from build123d import *

# Parameters (mm, degrees)
SKETCH1_W         = 247
SKETCH1_H         = 293
MAIN_BASE_DEPTH   = 3.175
HANDLES_DEPTH     = 192.715472772
ALIGNMENT_HOLES_D = 6.99999997


with BuildPart() as part:
    # Sketch1 → Main Base (new, symmetric)
    with BuildSketch(Plane(origin=(0, 0, 0), x_dir=(1, 0, 0), z_dir=(0, 1, 0))):
        Rectangle(SKETCH1_W, SKETCH1_H)
    extrude(amount=MAIN_BASE_DEPTH, both=True)

    # Sketch2 → Handles (cut, through all)
    with BuildSketch(Plane(origin=(0, 3.175, 0), x_dir=(1, 0, 0), z_dir=(0, 1, 0))):
        with BuildLine():
            Line((-38.1, 133.8), (38.1, 133.8))
            ThreePointArc((38.1, 133.8), (50.8, 121.1), (38.1, 108.4))
            Line((38.1, 108.4), (-38.1, 108.4))
            ThreePointArc((-38.1, 108.4), (-50.8, 121.1), (-38.1, 133.8))
        make_face()
        with BuildLine():
            Line((-38.1, -133.8), (38.1, -133.8))
            ThreePointArc((38.1, -133.8), (50.8, -121.1), (38.1, -108.4))
            Line((38.1, -108.4), (-38.1, -108.4))
            ThreePointArc((-38.1, -108.4), (-50.8, -121.1), (-38.1, -133.8))
        make_face()
    extrude(amount=-HANDLES_DEPTH, mode=Mode.SUBTRACT)

    # Alignment Holes (through all)
    with Locations(Plane(origin=(0, 3.175, 0), x_dir=(1, 0, 0), z_dir=(0, 1, 0))):
        with Locations((-106, 0), (-37, -39.837168574), (-37, 39.837168574), (37, 39.837168574), (37, -39.837168574), (106, 0)):
            Hole(ALIGNMENT_HOLES_D / 2)


solid = part.part
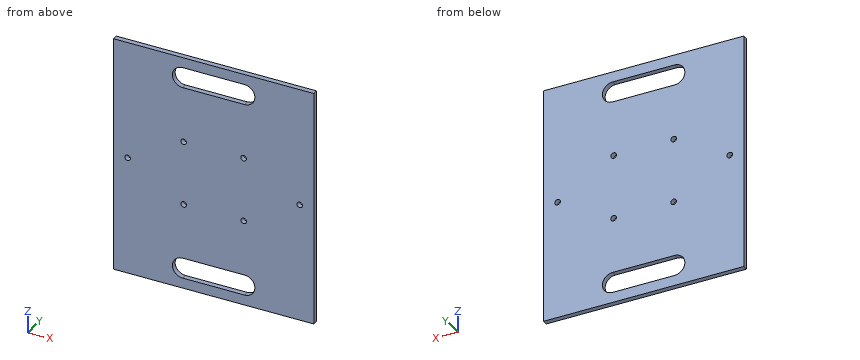
Can you work these out from the model? Positions are in its coordinate system, mm. Round coordinates to 2 decimals unless told otherwise and drop trailing zeros. Loops run counter-clockwise (first coordinate to the right, second up) from the corner with the lowest first, then second, coordinate; pieces in that order, holes last. Notation, with made-up numbers: (67.5, -7.5) - (80.5, -7.5) arc R9 ccw to (80.5, 0.5) - close; hole circle Ø1 at (33, 75). An arc over 180 degrees is marked (long way). Write item = value, one per line. Start each with the question number.
(1) If we section it at C-C (z = 0): Please give me the cut outline in (x, y) (3 decimals), and give its area (3 significant figures).
(2) If I drill on probe 1 along Z at (x, y) = (-28.5, 1.75); probe 2 along Z at (x, y) = (37, 0.25); probe 3 along Z at (x, y) = (45, 1.25), over which ranges is the centre line in solid material (lowest first)? Write a range as [from, to].
(3) If we section it at D-D (x = 19): Please give me the cut outline in (y, z) (3 decimals), and give its area (3 significant figures).
(4) For P1, Ø4, axis at x = -106, z = 0, coming from the +Y side; P2, Ø11, axis at x = 37, z = -39.84, coming from the +Y side (3 decimals), each with a flat end and sliding along its axis, tell me the tip position at first contact or that it passes through.
(5) If we section it at B-B (x = 106): Please give me the cut outline in (y, z) (3 decimals).
(6) If we section it at A-A (z = 121.1): Please give me the cut outline in (x, y) (3 decimals), and give its area (3 significant figures).
Ans:
q1.outline = (-123.5, -3.175) - (-109.5, -3.175) - (-109.5, 3.175) - (-123.5, 3.175) - close; (-102.5, -3.175) - (102.5, -3.175) - (102.5, 3.175) - (-102.5, 3.175) - close; (109.5, -3.175) - (123.5, -3.175) - (123.5, 3.175) - (109.5, 3.175) - close
q1.area = 1,480 mm²
q2.probe_1 = [-146.5, -133.8], [-108.4, 108.4], [133.8, 146.5]
q2.probe_2 = [-146.5, -133.8], [-108.4, -43.34], [-36.34, 36.34], [43.34, 108.4], [133.8, 146.5]
q2.probe_3 = [-146.5, -131.76], [-110.44, 110.44], [131.76, 146.5]
q3.outline = (-3.175, -146.5) - (3.175, -146.5) - (3.175, -133.8) - (-3.175, -133.8) - close; (-3.175, -108.4) - (3.175, -108.4) - (3.175, 108.4) - (-3.175, 108.4) - close; (-3.175, 133.8) - (3.175, 133.8) - (3.175, 146.5) - (-3.175, 146.5) - close
q3.area = 1,540 mm²
q4.P1 = through
q4.P2 = 3.175
q5.outline = (-3.175, -146.5) - (3.175, -146.5) - (3.175, -3.5) - (-3.175, -3.5) - close; (-3.175, 3.5) - (3.175, 3.5) - (3.175, 146.5) - (-3.175, 146.5) - close
q6.outline = (-123.5, -3.175) - (-50.8, -3.175) - (-50.8, 3.175) - (-123.5, 3.175) - close; (50.8, -3.175) - (123.5, -3.175) - (123.5, 3.175) - (50.8, 3.175) - close
q6.area = 923 mm²
